Autodesk Inventor part; units mm, degrees
ref_plane "YZ Plane" through (0, 0, 0) normal (1, 0, 0) x (0, 1, 0)
ref_plane "XZ Plane" through (0, 0, 0) normal (0, 1, 0) x (-1, 0, 0)
ref_plane "XY Plane" through (0, 0, 0) normal (0, 0, 1) x (1, 0, 0)
sketch "Sketch1" plane through (0, 0, 0) normal (0, 1, 0) x (-1, 0, 0)
  line L0 (6.6, 6.6) -> (-6.6, 6.6)
  line L1 (-6.6, 6.6) -> (-6.6, -6.6)
  line L2 (-6.6, -6.6) -> (6.6, -6.6)
  line L3 (6.6, -6.6) -> (6.6, 6.6)
  line L4 (6.6, 6.6) -> (-6.6, -6.6) construction
  line L5 (-6.6, 6.6) -> (6.6, -6.6) construction
  point P0 (0, 0)
  dimension "d0" = 13.2
extrude "Extrusion1" add sketch "Sketch1" along normal mid plane 13.2
sketch "Sketch2" plane through (0, 6.6, 0) normal (0, 1, 0) x (1, 0, 0)
  circle A0 centre (0, 0) radius 1.35
  dimension "d3" = 2.7
sketch "Sketch3" plane through (6.6, -6.6, -6.6) normal (1, 0, 0) x (0, 0, -1)
  circle A0 centre (-6.6, 6.6) radius 1.35
  dimension "d4" = 2.7
sketch "Sketch4" plane through (-6.6, 6.6, 6.6) normal (0, 0, 1) x (1, 0, 0)
  circle A0 centre (6.6, -6.6) radius 1.35
  dimension "d5" = 2.7
extrude "Extrusion2" cut sketch "Sketch4" along normal through all both and the other way through all
extrude "Extrusion3" cut sketch "Sketch2" along normal through all both and the other way through all
extrude "Extrusion4" cut sketch "Sketch3" against normal through all
equation "\"d1\" = d0"
equation "\"d4\" = d3"
equation "\"d5\" = d3"
properties part number "C-M3-M" material "ABS Plastic"
CAD build for the part. Positions are in the model's coordinates, mm. Coordinates: 2 decimals unless noted, no trailing zeros. Write each loop counter-clockwise with the first axis right and the second up, starting at its lowest first coordinate (ties: lowest second). Pieces come first, ordered by that corner, then holes. Notation, with made-up numbers: M 78,27 L 133,27 A19 ccw 133,37 Z; hole C -21.75,75 d2. An arc over 180 degrees is marked long. Return JSON: item names as keys, results as strings.
Item 1: Probe line 1 (X direction, y = 0, z = 4.55). List the from-to ranges inside material, lowest first. Write a range as from..to.
Findings below:
{"line 1": "x = -6.6..-1.35, 1.35..6.6"}
Item 2: Slice it at C-C, the plane z = 3.25. Write the cut outline in (x, y).
Findings below:
{"outline": "M -6.6,-6.6 L 6.6,-6.6 L 6.6,6.6 L -6.6,6.6 Z; hole C 0,0 d2.7"}
Item 3: Two-plate mould, pull along Y, no slides. Class faces 1 (the flat face through (0, -6.6, 2)), 2 (the flat face through (0, 6.6, 2)), 3 (the cylindrical face through (-3.74, 0.06, 1.35)), 4 (the cylindrical face through (-1.35, -3.74, -0.06)): +Y half, -Y half, draft (parallel to the pull), parting line (faces both ways), or undercut.
Findings below:
{"face 1": "-Y half", "face 2": "+Y half", "face 3": "undercut", "face 4": "draft"}
Item 4: Slice it at A-A, the plane z = 0. Write the cut outline in (x, y).
Findings below:
{"outline": "M -6.6,-6.6 L -1.35,-6.6 L -1.35,-1.35 L -6.6,-1.35 Z; M -6.6,1.35 L -1.35,1.35 L -1.35,6.6 L -6.6,6.6 Z; M 1.35,-6.6 L 6.6,-6.6 L 6.6,-1.35 L 1.35,-1.35 Z; M 1.35,1.35 L 6.6,1.35 L 6.6,6.6 L 1.35,6.6 Z"}
